```python
from build123d import *

# Parameters (mm, degrees)
F0_R     = 25.4
F1_DEPTH = 127
F1_TAPER = 3
F2_R     = 9.525
F3_SIZE  = 12.7
F4_W     = 13.4048998849
F4_H     = 5.8565368653
F5_DEPTH = 127.001


with BuildPart() as f1:
    # F0 (on Front) → F1 (new body)
    with BuildSketch(Plane.XZ):
        Circle(F0_R)
    extrude(amount=F1_DEPTH, taper=F1_TAPER)

    # F2
    f2_edges = [f1.edges().sort_by_distance(p)[0] for p in [
        (-18.744212, -127, 0),
    ]]
    fillet(f2_edges, radius=F2_R)

    # F3
    f3_edges = [f1.edges().sort_by_distance(p)[0] for p in [
        (-25.4, 0, 0),
    ]]
    chamfer(f3_edges, length=F3_SIZE)

    # F4 (on face) → F5 (cut, through all)
    with BuildSketch(Plane.XZ.offset(127)):
        with Locations((1.0366908521, -2.9282684326)):
            Rectangle(F4_W, F4_H)
    extrude(amount=-F5_DEPTH, mode=Mode.SUBTRACT)


solid = f1.part
```
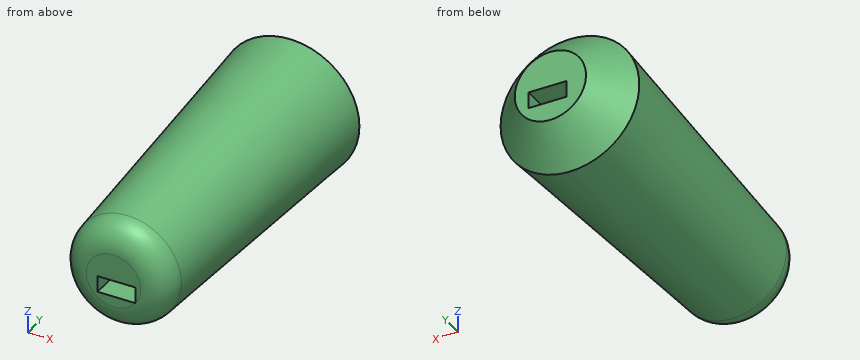
Input: part model. Units: mm. Frame: model coordinates. Round coordinates to 2 decimals unless told otherwise and drop trailing zeros. Order: outer loops, then holes, each group sorted by start corner. A loop starts at its lowest first (then second) coordinate and runs counter-clockwise, first axis right, second up. Notation, with made-up numbers: (-26, 73.25) - (13, 73.25) arc R33 ccw to (13, 104.25) - close; hole circle Ø4 at (-0.5, 65). An arc over 180 degrees is marked (long way). Answer in a Markdown table with one row per item.
Item 1: Pin query (flat end, axial travel): pin 1 (10 mm diameter, centred on x = 0.5, y = -60, fed in from -Z); pin 2 (6.5 mm diameter, centred on x = 2, y = -44, fed in from +Z); pin 3 (2 mm diameter, centred on y = -111.5, z = 4, fed in from +X). Return the tip coordinate at first contact, or that it passes through.
Model answer:
| item | result |
|---|---|
| pin 1 | stops at z = -22.52 |
| pin 2 | stops at z = 23.24 |
| pin 3 | stops at x = 19.33 |
Item 2: Line query: line 1 (Z direction, x = 7, y = -89); line 2 (X direction, y = -55, z = -2); line 3 (Z direction, x = 0, y = -47). Output: solid intervals per line, ascending.
Model answer:
| item | result |
|---|---|
| line 1 | z = -19.52 to -5.86, 0 to 19.52 |
| line 2 | x = -22.43 to -5.67, 7.74 to 22.43 |
| line 3 | z = -22.94 to -5.86, 0 to 22.94 |
Item 3: Section query B-B (y = -96). Return the cut outline in (x, z), then the cut area to 3 significant figures.
Model answer:
| item | result |
|---|---|
| outline | circle Ø40.74 at (0, 0); hole (-5.67, -5.86) - (7.74, -5.86) - (7.74, 0) - (-5.67, 0) - close |
| area | 1,220 mm² |
Item 4: Section query C-C (y = -67.5). Return the cut outline in (x, z), then the cut area to 3 significant figures.
Model answer:
| item | result |
|---|---|
| outline | circle Ø43.72 at (0, 0); hole (-5.67, -5.86) - (7.74, -5.86) - (7.74, 0) - (-5.67, 0) - close |
| area | 1,420 mm² |
